CAD build for the part. Positions are in the model's coordinates, mm. Face numbers are marked on the shaded views. Coordinates: 2 decimals unless noted, no trailing zeros. Loops run counter-clockwise (first coordinate to the right, second up) from the corner with the lowest first, then second, coordinate; pieces in that order, holes last.
1) Wall check: line 1 along Z through (x, y) = (10, -22); line 2 along Z through (x, y) = (20, 34); line 3 along Z through (x, y) = (29.5, 13). Give the ranges that are in metal, low to high.
2) Two-plate mould, pull along Z, no slides. Class the marked faces 1, 2 and 3: +Z half, -Z half, draft (parallel to the pull), parting line (faces both ways), or undercut.
3) Pin check, flat tips, straight feed: pin 1 Ø1 at (x, y) = (18, 38.5) entering from -Z; pin 2 Ø3 at (x, y) = (21, 40.5) entering from -Z. Stop position of each tip, or through.
4) Saw through at A-A, the plane y = 33.5. Give the number of separate pieces and of enclosed holes in the cut face, and give its area (3 significant figures).
5) Saw through at C-C, the plane z = -1.75. Write the cut outline in (x, y) (3 decimals).
```python
from build123d import *

# Parameters (mm, degrees)
F0_R     = 31.75
F1_DEPTH = 12.7
F5_DEPTH = 6.35
F7_DEPTH = 6.35
F8_SIZE  = 3.17499


# Not quite as in the source:
# - a fillet or chamfer is up to 0.001 mm smaller than in the source, because OpenCascade refuses the exact size


with BuildPart() as f1:
    # F0 (on Top) → F1 (new body, symmetric)
    with BuildSketch(Plane.XY):
        Circle(F0_R)
    extrude(amount=F1_DEPTH, both=True)

    # F2 (on Front) → F3 (revolve, cut)
    with BuildSketch(Plane.XZ):
        Polygon((31.75, 6.35), (15.875, 6.35), (15.875, -6.35), (31.75, -6.35), (33.2811660987, -6.35), (33.2811660987, 6.35), align=None)
    revolve(axis=Axis((0, 0, 3.175), (0, 0, 1)), mode=Mode.SUBTRACT)

    # F4 (on face) → F5 (join)
    with BuildSketch(Plane.XY.offset(12.7)):
        with BuildLine():
            ThreePointArc((0, 31.75), (6.3734153916, 31.1037309056), (12.487369908, 29.1912331494))
            Line((12.487369908, 29.1912331494), (0, 63.5))
            Line((0, 63.5), (0, 31.75))
        make_face()
        with BuildLine():
            ThreePointArc((-12.487369908, 29.1912331494), (-6.3734153916, 31.1037309056), (0, 31.75))
            Line((0, 31.75), (0, 63.5))
            Line((0, 63.5), (-12.487369908, 29.1912331494))
        make_face()
        with BuildLine():
            ThreePointArc((-31.621322022, -2.8556073925), (-30.1960443924, 9.8112895714), (-23.9037029888, 20.8967816523))
            Line((-23.9037029888, 20.8967816523), (-60.3920887847, 19.6225791428))
            Line((-60.3920887847, 19.6225791428), (-31.621322022, -2.8556073925))
        make_face()
        with BuildLine():
            Line((-37.3243635206, -51.3725791428), (-7.0556818708, -30.9560955764))
            ThreePointArc((-7.0556818708, -30.9560955764), (-18.6621817603, -25.6862895714), (-27.2606708121, -16.2763118327))
            Line((-27.2606708121, -16.2763118327), (-37.3243635206, -51.3725791428))
        make_face()
        with BuildLine():
            Line((37.3243635206, -51.3725791428), (27.2606708121, -16.2763118327))
            ThreePointArc((27.2606708121, -16.2763118327), (18.6621817603, -25.6862895714), (7.0556818708, -30.9560955764))
            Line((7.0556818708, -30.9560955764), (37.3243635206, -51.3725791428))
        make_face()
        with BuildLine():
            ThreePointArc((23.9037029888, 20.8967816523), (29.7237705372, 11.160643577), (31.75, 0))
            ThreePointArc((31.75, 0), (31.7178141917, -1.4292525671), (31.621322022, -2.8556073925))
            Line((31.621322022, -2.8556073925), (60.3920887847, 19.6225791428))
            Line((60.3920887847, 19.6225791428), (23.9037029888, 20.8967816523))
        make_face()
    extrude(amount=-F5_DEPTH)

    # F6 (on face) → F7 (join)
    with BuildSketch(Plane(origin=(0, 0, -12.7), x_dir=(1, 0, 0), z_dir=(0, 0, -1))):
        with BuildLine():
            ThreePointArc((-12.487369908, 29.1912331494), (-6.3734153916, 31.1037309056), (0, 31.75))
            Line((0, 31.75), (0, 63.5))
            Line((0, 63.5), (-12.487369908, 29.1912331494))
        make_face()
        with BuildLine():
            ThreePointArc((0, 31.75), (6.3734153916, 31.1037309056), (12.487369908, 29.1912331494))
            Line((12.487369908, 29.1912331494), (0, 63.5))
            Line((0, 63.5), (0, 31.75))
        make_face()
        with BuildLine():
            ThreePointArc((-31.621322022, -2.8556073925), (-30.1960443924, 9.8112895714), (-23.9037029888, 20.8967816523))
            Line((-23.9037029888, 20.8967816523), (-60.3920887847, 19.6225791428))
            Line((-60.3920887847, 19.6225791428), (-31.621322022, -2.8556073925))
        make_face()
        with BuildLine():
            ThreePointArc((23.9037029888, 20.8967816523), (29.7237705372, 11.160643577), (31.75, 0))
            ThreePointArc((31.75, 0), (31.7178141917, -1.4292525671), (31.621322022, -2.8556073925))
            Line((31.621322022, -2.8556073925), (60.3920887847, 19.6225791428))
            Line((60.3920887847, 19.6225791428), (23.9037029888, 20.8967816523))
        make_face()
        with BuildLine():
            Line((-37.3243635206, -51.3725791428), (-7.0556818708, -30.9560955764))
            ThreePointArc((-7.0556818708, -30.9560955764), (-18.6621817603, -25.6862895714), (-27.2606708121, -16.2763118327))
            Line((-27.2606708121, -16.2763118327), (-37.3243635206, -51.3725791428))
        make_face()
        with BuildLine():
            Line((37.3243635206, -51.3725791428), (27.2606708121, -16.2763118327))
            ThreePointArc((27.2606708121, -16.2763118327), (18.6621817603, -25.6862895714), (7.0556818708, -30.9560955764))
            Line((7.0556818708, -30.9560955764), (37.3243635206, -51.3725791428))
        make_face()
    extrude(amount=-F7_DEPTH)

    # F8 (size 3.175 in the source; OpenCascade refuses exactly that, so slightly less here)
    f8_edges = [f1.edges().sort_by_distance(p)[0] for p in [
        (18.662182, 25.68629, 12.7),
        (6.243685, 46.345617, 12.7),
        (-6.243685, 46.345617, 12.7),
        (-18.662182, 25.68629, 12.7),
        (-42.147896, 20.25968, 12.7),
        (-46.006705, 8.383486, 12.7),
        (-30.196044, -9.81129, 12.7),
        (-32.292517, -33.824445, 12.7),
        (-22.190023, -41.164337, 12.7),
        (0, -31.75, 12.7),
        (22.190023, -41.164337, 12.7),
        (32.292517, -33.824445, 12.7),
        (30.196044, -9.81129, 12.7),
        (46.006705, 8.383486, 12.7),
        (42.147896, 20.25968, 12.7),
        (30.196044, 9.81129, -6.35),
        (46.006705, -8.383486, -6.35),
        (42.147896, -20.25968, -6.35),
        (18.662182, -25.68629, -6.35),
        (6.243685, -46.345617, -6.35),
        (-6.243685, -46.345617, -6.35),
        (-18.662182, -25.68629, -6.35),
        (-42.147896, -20.25968, -6.35),
        (-46.006705, -8.383486, -6.35),
        (-30.196044, 9.81129, -6.35),
        (-32.292517, 33.824445, -6.35),
        (-22.190023, 41.164337, -6.35),
        (0, 31.75, -6.35),
        (22.190023, 41.164337, -6.35),
        (32.292517, 33.824445, -6.35),
        (-15.875, 0, -6.35),
        (18.662182, 25.68629, 6.35),
        (6.243685, 46.345617, 6.35),
        (-6.243685, 46.345617, 6.35),
        (-18.662182, 25.68629, 6.35),
        (-42.147896, 20.25968, 6.35),
        (-46.006705, 8.383486, 6.35),
        (-30.196044, -9.81129, 6.35),
        (-32.292517, -33.824445, 6.35),
        (-22.190023, -41.164337, 6.35),
        (0, -31.75, 6.35),
        (22.190023, -41.164337, 6.35),
        (32.292517, -33.824445, 6.35),
        (30.196044, -9.81129, 6.35),
        (46.006705, 8.383486, 6.35),
        (42.147896, 20.25968, 6.35),
        (-15.875, 0, 6.35),
        (30.196044, 9.81129, -12.7),
        (32.292517, 33.824445, -12.7),
        (22.190023, 41.164337, -12.7),
        (0, 31.75, -12.7),
        (-22.190023, 41.164337, -12.7),
        (-32.292517, 33.824445, -12.7),
        (-30.196044, 9.81129, -12.7),
        (-46.006705, -8.383486, -12.7),
        (-42.147896, -20.25968, -12.7),
        (-18.662182, -25.68629, -12.7),
        (-6.243685, -46.345617, -12.7),
        (6.243685, -46.345617, -12.7),
        (18.662182, -25.68629, -12.7),
        (42.147896, -20.25968, -12.7),
        (46.006705, -8.383486, -12.7),
    ]]
    chamfer(f8_edges, length=F8_SIZE)


solid = f1.part
```
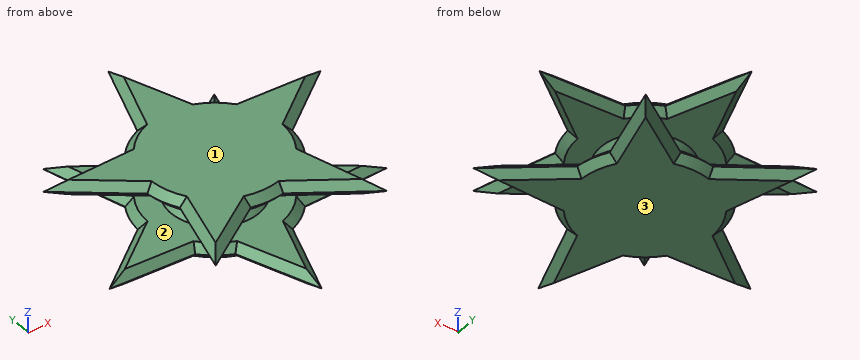
Data:
1. line 1: z = -12.7 to -6.35, 6.35 to 12.7
1. line 2: z = -12.7 to -6.35
1. line 3: z = 6.35 to 12.7
2. face 1: +Z half
2. face 2: undercut
2. face 3: -Z half
3. pin 1: stops at z = -9.89
3. pin 2: stops at z = -10.91
4. separate pieces: 3
4. enclosed holes: 0
4. area: 332 mm2
5. outline: circle Ø31.75 at (0, 0)
